Autodesk Inventor part; units mm, degrees
ref_plane "YZ Plane" through (0, 0, 0) normal (1, 0, 0) x (0, 1, 0)
ref_plane "XZ Plane" through (0, 0, 0) normal (0, 1, 0) x (-1, 0, 0)
ref_plane "XY Plane" through (0, 0, 0) normal (0, 0, 1) x (1, 0, 0)
sketch "Skizze1" plane through (0, 0, 0) normal (0, 0, 1) x (1, 0, 0)
  circle A0 centre (0, 0) radius 3
  dimension "d0" = 6
extrude "Extrusion1" add sketch "Skizze1" along normal blind 24
sketch "Skizze2" plane through (0, 0, 0) normal (0, 0, -1) x (-1, 0, 0)
  point P0 (0, 0)
hole "Bohrung1" at (0, 0, 0) direction (0, 0, 1) diameter 1.2 end through all
sketch "Skizze3" plane through (0, 0, 24) normal (0, 0, 1) x (1, 0, 0)
  point P0 (0, 0)
hole "Bohrung2" at (0, 0, 24) direction (0, 0, -1) diameter 2.4 depth 10 tip angle 118
chamfer "Fase1" distance 1.6 angle 45 1 edges at (0, 1.2, 24)
properties part number "PTFE - Isolator" material "Polytetrafluoroethylen"
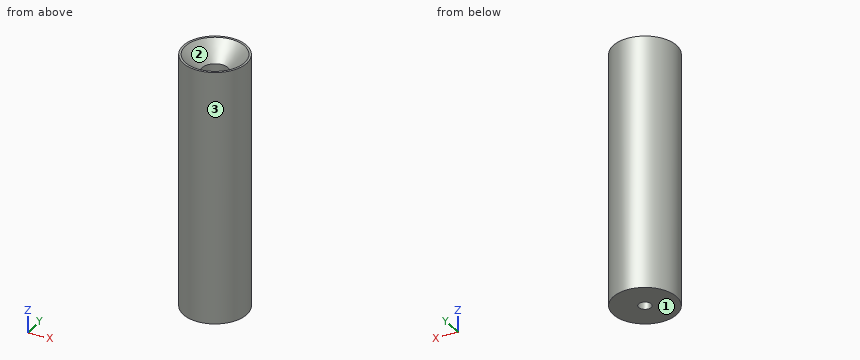
For this review, take the finished solid that the model builds, in its own axes (mm). Face numbers are marked on the shaded views. Round coordinates to 2 decimals unless told otherwise and drop trailing zeros. Write each loop counter-clockwise with the first axis right and the second up, starting at its lowest first coordinate (ties: lowest second). Pieces come first, ordered by that corner, then holes. Notation, with made-up numbers: (40.25, 8) -> (95.25, 8) arc R7 cw to (95.25, 21) -> close; hole circle Ø9 at (-23, 64). An arc over 180 degrees is marked (long way). Use one line per item in the form item = value.
1) Clearance check with flat-ended pins moving along their axes: pin 1 (2 mm diameter, centred on x = 0, y = 0, fed in from +Z); pin 2 (1 mm diameter, centred on y = 1, z = 10.5, fed in from +X); pin 3 (1.4 mm diameter, centred on x = 0, y = 0, fed in from +Z). State where each tip first meets the part, or that it passes through.
Found:
pin_1 = 13.88
pin_2 = 2.96
pin_3 = 13.7
2) Take a section at D-D, the plane z = 7.25. Write out the cut boundary in (x, y).
Found:
outline = circle Ø6 at (0, 0); hole circle Ø1.2 at (0, 0)
3) Take a section at C-C, the plane z = 18.75. Write out the cut boundary in (x, y).
Found:
outline = circle Ø6 at (0, 0); hole circle Ø2.4 at (0, 0)
4) To check wall thickness, follow L1, parallel to Y at x = 0, z = 8.5; L2, parallel to Y at x = -0.4, z = 1.75; L3, parallel to X at y = 0.35, z = 6. State the ranges of each line that lie inside material, in increasing order. Write a range as from..to.
Found:
L1 = -3..-0.6, 0.6..3
L2 = -2.97..-0.45, 0.45..2.97
L3 = -2.98..-0.49, 0.49..2.98
5) Mouldability with a two-part tool opening along X and no side actions: class the marked faces 1, 2 and 3 as +X half, -X half, draft (parallel to the pull), parting line (faces both ways), or undercut.
Found:
face_1 = draft
face_2 = undercut
face_3 = parting line
6) Take a section at A-A, the plane x = 0. Write out the cut boundary in (y, z), and give its area (3 significant figures).
Found:
outline = (-3, 0) -> (-0.6, 0) -> (-0.6, 13.64) -> (-1.2, 14) -> (-1.2, 22.4) -> (-2.8, 24) -> (-3, 24) -> close; (0.6, 0) -> (3, 0) -> (3, 24) -> (2.8, 24) -> (1.2, 22.4) -> (1.2, 14) -> (0.6, 13.64) -> close
area = 100 mm2
